Source: CAD feature listing. Evaluate the final solid. Frame: model axes, mm. Give positions to 0.01 mm unless a question says otherwise; leave off trailing zeros. Write each loop counter-clockwise with the first axis right and the second up, starting at its lowest first coordinate (ties: lowest second). Pieces come first, ordered by that corner, then holes. Notation, with made-up numbers: (-11, -3.75) -> (44, -3.75) arc R19 cw to (44, 21.25) -> close; hole circle Ø8 at (13.5, -23). An arc over 180 degrees is marked (long way). Write item = value, one per line.
from build123d import *

# Parameters (mm, degrees)
SKETCH_W        = 165
SKETCH_H        = 92
PAD_DEPTH       = 2
SKETCH001_W     = 21
SKETCH001_H     = 90
POCKET_DEPTH    = 5
SKETCH002_R     = 4
POCKET001_DEPTH = 5
SKETCH003_W     = 40
SKETCH003_H     = 60
POCKET002_DEPTH = 5
SKETCH004_R     = 8.5
POCKET003_DEPTH = 5
SKETCH005_W     = 70
SKETCH005_H     = 30
POCKET004_DEPTH = 5


with BuildPart() as part:
    # Sketch → Pad (new body)
    with BuildSketch(Plane.XY):
        Rectangle(SKETCH_W, SKETCH_H)
    extrude(amount=PAD_DEPTH)

    # Sketch001 → Pocket (cut)
    with BuildSketch(Plane.XY):
        with Locations((-30.5, 0)):
            Rectangle(SKETCH001_W, SKETCH001_H)
    extrude(amount=POCKET_DEPTH, mode=Mode.SUBTRACT)

    # Sketch002 → Pocket001 (cut)
    with BuildSketch(Plane.XY):
        with Locations((-4.5, 29)):
            Circle(SKETCH002_R)
        with Locations((13, 29)):
            Circle(SKETCH002_R)
        with Locations((30.5, 29)):
            Circle(SKETCH002_R)
        with Locations((48, 29)):
            Circle(SKETCH002_R)
        with Locations((65.5, 29)):
            Circle(SKETCH002_R)
    extrude(amount=POCKET001_DEPTH, mode=Mode.SUBTRACT)

    # Sketch003 → Pocket002 (cut)
    with BuildSketch(Plane.XY):
        with Locations((-61.75, -15.25)):
            Rectangle(SKETCH003_W, SKETCH003_H)
    extrude(amount=POCKET002_DEPTH, mode=Mode.SUBTRACT)

    # Sketch004 → Pocket003 (cut)
    with BuildSketch(Plane.XY):
        with Locations((-62.5, 31)):
            Circle(SKETCH004_R)
    extrude(amount=POCKET003_DEPTH, mode=Mode.SUBTRACT)

    # Sketch005 → Pocket004 (cut)
    with BuildSketch(Plane.XY):
        with Locations((32.5, -21)):
            Rectangle(SKETCH005_W, SKETCH005_H)
    extrude(amount=POCKET004_DEPTH, mode=Mode.SUBTRACT)


solid = part.part
1) Cut plane C-C (z = 1.5). State how many separate pieces and enclosed holes the cut face has, then the cut area to 3 significant figures.
Computed:
separate_pieces = 1
enclosed_holes = 9
area = 8,310 mm²
2) Cut plane B-B (x = 30.5). Return the cut outline in (y, z), then the cut area to 3 significant figures.
Computed:
outline = (-46, 0) -> (-36, 0) -> (-36, 2) -> (-46, 2) -> close; (-6, 0) -> (25, 0) -> (25, 2) -> (-6, 2) -> close; (33, 0) -> (46, 0) -> (46, 2) -> (33, 2) -> close
area = 108 mm²
3) Cut plane A-A (x = -48). Return the cut outline in (y, z), then the cut area to 3 significant figures.
Computed:
outline = (-46, 0) -> (-45.25, 0) -> (-45.25, 2) -> (-46, 2) -> close; (14.75, 0) -> (46, 0) -> (46, 2) -> (14.75, 2) -> close
area = 64.0 mm²
4) Draft query along Y for faces 1 (the flat face through (17, 11, 0)), 2 (the cylindrical face through (29.979, 32.966, 0.986)), 3 (the cylindrical face through (12.479, 32.966, 0.986)). Return one class per face: pulls with the +Y half, pulls with the -Y half, needs draft (parallel to the pull), parting line crosses it, or undercut.
Computed:
face_1 = needs draft
face_2 = undercut
face_3 = undercut
5) Contact query for a flat-ended pin moving along its axis: pin 1 (7 mm diameter, centred on x = 48, y = 29, fed in from -Z). Output: stop coordinate, or through.
Computed:
pin_1 = through
6) Material intervals for L1, parallel to X at y = 10, z = 1.2; L2, parallel to X at y = -33, z = 1.65; L3, parallel to Y at x = 13, z = 0.9, sorted ascending.
Computed:
L1 = -82.5 to -81.75, -41.75 to -41, -20 to 82.5
L2 = -82.5 to -81.75, -41.75 to -41, -20 to -2.5, 67.5 to 82.5
L3 = -46 to -36, -6 to 25, 33 to 46
